Read the model definition and answer for the solid it produces. Units are mm, in the model's axes. A direction names the side the tool comes from. Coordinates: 2 decimals unless noted, no trailing zeros. Order: outer loops, then holes, each group sorted by start corner. A loop starts at its lowest first (then second) coordinate and runs counter-clockwise, first axis right, second up. Notation, with made-up numbers: (45.5, 36.5) -> (55.5, 36.5) arc R35 cw to (55.5, 74.5) -> close; hole circle Ø5 at (-4.5, 51). An arc over 180 degrees is marked (long way). Answer as a JSON object with one key per item and string values. Group by question number.
1) Consider L1, parallel to Z at x = 2.5, y = 8.5; L2, parallel to X at y = 3.75, z = -0.25; L3, parallel to X at y = 4, z = 2. Determine where each line is inside the solid, lowest interval first.
2) A tool of negligible diameter and unlimited length cuts with its end or side. For faces 5 (the cylindrical face through (7.197, 6.084, 4.859)), 6 (the flat face through (0, 6, -5.5)), 7 (the flat face through (-2.65, 6, 1)), from which of +Z, -Z, +X, -X, +Y, -Y can it reach the whole face along a straight path? Write none if from no direction.
3) Section B-B on y = 10 is taken. Determine the outline of the cut face in (x, z), and give its area (3 significant figures).
4) Given pin 1 (6 mm diameter, centred on y = 5.5, z = 4, fed in from +X), flat-ended and moving along its own axis, determine where the tip first touches the part or whether it passes through.
5) Section D-D on z = 3 is taken. Determine the outline of the cut face in (x, y), and give its area (3 significant figures).
6) Section A-A on z = 0.5 is taken. Determine the outline of the cut face in (x, y), and give its area (3 significant figures).
7) Section C-C on x = -4.75 is taken. Determine the outline of the cut face in (y, z), and give its area (3 significant figures).
8) Determine the mould class of faces 1 (the flat face through (0, 12, 3)), 2 (the flat face through (-2, 4, -5.5)), 3 (the flat face through (-4, 6, 0)), 4 (the flat face through (2, 8, -5.5)) for opening direction Y: released by +Y, released by -Y, zero draft, split by the parting line, or undercut.
Autodesk Inventor part; units mm, degrees
ref_plane "YZ Plane" through (0, 0, 0) normal (1, 0, 0) x (0, 1, 0)
ref_plane "XZ Plane" through (0, 0, 0) normal (0, 1, 0) x (-1, 0, 0)
ref_plane "XY Plane" through (0, 0, 0) normal (0, 0, 1) x (1, 0, 0)
sketch "Skizze1" plane through (0, 0, 0) normal (0, 1, 0) x (-1, 0, 0)
  line L0 (-5.15, 2.75) -> (2.65, 2.75)
  line L1 (2.65, 2.75) -> (2.65, 0)
  line L2 (2.65, 0) -> (5.15, 0)
  line L3 (5.15, 0) -> (5.15, -2.75)
  line L4 (5.15, -2.75) -> (-5.15, -2.75)
  line L5 (-5.15, -2.75) -> (-5.15, 2.75)
  line L6 (8.4, 6) -> (-8.4, 6)
  line L7 (-8.4, 6) -> (-8.4, -6)
  line L8 (-8.4, -6) -> (8.4, -6)
  line L9 (8.4, -6) -> (8.4, 6)
  line L10 (8.4, 6) -> (-8.4, -6) construction
  line L11 (-8.4, 6) -> (8.4, -6) construction
  point P0 (0, 0)
  point P1 (0, 0)
  dimension "d0" = 16.8
  dimension "d1" = 12
  dimension "d2" = 5.5
  dimension "d3" = 10.3
  dimension "d4" = 2.75
  dimension "d5" = 7.8
  dimension "d6" = 2.75
  dimension "d7" = 3.25
  dimension "d8" = 3.25
extrude "Extrusion1" add sketch "Skizze1" along normal blind 12
fillet "Rundung1" radius 4 4 edges at (8.4, 6, -6) (8.4, 6, 6) (-8.4, 6, -6) (-8.4, 6, 6)
sketch "Skizze3" plane through (4.4, 0, -6) normal (0, 0, -1) x (-1, 0, 0)
  line L0 (8.075, 6) -> (6.525, 6)
  line L1 (6.525, 6) -> (4.3724, 2.7478)
  line L2 (8.075, 6) -> (5.9224, 2.7478)
  line L3 (8.075, 6) -> (11.975, 6) construction
  line L4 (5.9224, 2.7478) -> (4.3724, 2.7478)
  line L5 (3.0224, 2.7478) -> (7.3276, 9.2522)
  line L6 (3.0224, 2.7478) -> (10.8224, 2.7478) construction
  line L7 (7.3276, 9.2522) -> (5.7776, 9.2522)
  line L8 (7.3276, 9.2522) -> (8.8776, 9.2522) construction
  line L9 (5.7776, 9.2522) -> (1.4724, 2.7478)
  line L10 (1.4724, 2.7478) -> (3.0224, 2.7478)
  line L11 (4.4276, 9.2522) -> (2.8776, 9.2522)
  line L12 (2.8776, 9.2522) -> (0.725, 6)
  line L13 (0.725, 6) -> (2.275, 6)
  line L14 (0.725, 6) -> (2.275, 6) construction
  line L15 (2.275, 6) -> (4.4276, 9.2522)
  line L16 (-4, 12) -> (-4, 0)
  line L17 (12.8, 0) -> (12.8, 12)
  line L18 (0, 12) -> (8.8, 12)
  line L19 (0, 0) -> (8.8, 0)
  point P0 (4.4, 0)
  point P1 (0, 12.9522)
  dimension "d21" = 3.9
  dimension "d22" = 123.5
  dimension "d23" = 3.9
  dimension "d24" = 123.5
  dimension "d25" = 7.8
  dimension "d26" = 56.5
  dimension "d27" = 1.55
  dimension "d28" = 1.55
  dimension "d29" = 1.55
  dimension "d30" = 180
  dimension "d31" = 123.5
  dimension "d32" = 1.55
  dimension "d33" = 3.9
  dimension "d34" = 123.5
  dimension "d35" = 1.55
  dimension "d36" = 0
  dimension "d37" = 1.35
  dimension "d38" = 1.35
  dimension "d39" = 7.35
  dimension "d42" = 3.7
  dimension "d43" = 0
  dimension "d50" = 4.725
  dimension "d51" = 4.725
  dimension "d52" = 2.7479
  dimension "d53" = 2.7479
extrude "Extrusion3" cut sketch "Skizze3" against normal blind 0.5
chamfer "Fase2" distance 0.5 angle 45 6 edges at (-2.1526, 9.2522, -5.5) (-2.9, 6, -5.5) (0.7474, 9.2522, -5.5) (2.9, 6, -5.5) (2.1526, 2.7478, -5.5) (-0.7474, 2.7478, -5.5)
equation "\"d0\" = d3 + 2 * d7"
equation "\"d7\" = d8"
equation "\"d37\" = d38"
equation "\"d50\" = d51"
equation "\"d52\" = d53"
properties part number "Plugholder"
Worked answers:
{
 "1": {"L1": "z = -6 to -2.75, 2.75 to 6", "L2": "x = -8.4 to -5.15, 5.15 to 8.4", "L3": "x = -8.4 to -2.65, 5.15 to 8.4"},
 "2": {"face 5": "+Z, +X, +Y, -Y", "face 6": "-Z", "face 7": "+Y, -Y"},
 "3": {"outline": "(-8.4, -2) arc R4 ccw to (-4.4, -6) -> (4.4, -6) arc R4 ccw to (8.4, -2) -> (8.4, 2) arc R4 ccw to (4.4, 6) -> (-4.4, 6) arc R4 ccw to (-8.4, 2) -> close; hole (-5.15, -2.75) -> (5.15, -2.75) -> (5.15, 2.75) -> (-2.65, 2.75) -> (-2.65, 0) -> (-5.15, 0) -> close", "area": "138 mm²"},
 "4": {"pin 1": "stops at x = 8.4"},
 "5": {"outline": "(-8.27, 0) -> (8.27, 0) -> (8.27, 12) -> (-8.27, 12) -> close", "area": "199 mm²"},
 "6": {"outline": "(-8.4, 0) -> (-2.65, 0) -> (-2.65, 12) -> (-8.4, 12) -> close; (5.15, 0) -> (8.4, 0) -> (8.4, 12) -> (5.15, 12) -> close", "area": "108 mm²"},
 "7": {"outline": "(0, -5.98) -> (12, -5.98) -> (12, -2.75) -> (0, -2.75) -> close; (0, 0) -> (12, 0) -> (12, 5.98) -> (0, 5.98) -> close", "area": "111 mm²"},
 "8": {"face 1": "released by +Y", "face 2": "undercut", "face 3": "zero draft", "face 4": "undercut"}
}
